from build123d import *

# Parameters (mm, degrees)
BOSS_EXTRUDE2_DEPTH  = 14.375
M4_CLEARANCE_HOLE2_D = 4.5
CUT_EXTRUDE1_START   = -5
SKETCH10_R           = 4.25
CUT_EXTRUDE1_DEPTH   = 30
M4_CLEARANCE_HOLE3_D = 4.5
CUT_EXTRUDE2_START   = -5
SKETCH14_R           = 4.25
CUT_EXTRUDE2_DEPTH   = 30
CHAMFER1_SIZE        = 1
FILLET2_R            = 1


with BuildPart() as part:
    # Sketch5 → Boss-Extrude2 (new, symmetric)
    with BuildSketch(Plane.XY):
        Polygon((0, 0), (0, 25.4), (-50.8, 0), align=None)
    extrude(amount=BOSS_EXTRUDE2_DEPTH, both=True)

    # M4 Clearance Hole2 (through all)
    with Locations(Plane(origin=(0, 0, 0), x_dir=(0, 0, -1), z_dir=(1, 0, 0))):
        with Locations((0, 12.390983006)):
            Hole(M4_CLEARANCE_HOLE2_D / 2)

    # Sketch10 → Cut-Extrude1 (cut)
    with BuildSketch(Plane(origin=(0, 0, 0), x_dir=(0, 0, -1), z_dir=(1, 0, 0)).offset(CUT_EXTRUDE1_START)):
        with Locations((0, 12.390983006)):
            Circle(SKETCH10_R)
    extrude(amount=-CUT_EXTRUDE1_DEPTH, mode=Mode.SUBTRACT)

    # M4 Clearance Hole3 (through all)
    with Locations(Plane(origin=(0, 0, 0), x_dir=(-1, 0, 0), z_dir=(0, -1, 0))):
        with Locations((25.4, 0)):
            Hole(M4_CLEARANCE_HOLE3_D / 2)

    # Sketch14 → Cut-Extrude2 (cut)
    with BuildSketch(Plane.XZ.offset(CUT_EXTRUDE2_START)):
        with Locations(Location((-25.4, 0, 0), (0, 0, 270))):
            Circle(SKETCH14_R)
    extrude(amount=-CUT_EXTRUDE2_DEPTH, mode=Mode.SUBTRACT)

    # Chamfer1
    chamfer1_edges = [part.edges().sort_by_distance(p)[0] for p in [
        (0, 0, 0),
    ]]
    chamfer(chamfer1_edges, length=CHAMFER1_SIZE)

    # Fillet2
    fillet2_edges = [part.edges().sort_by_distance(p)[0] for p in [
        (-25.4, 12.7, 14.375),
        (-25.4, 12.7, -14.375),
        (-25.9, 0, -14.375),
        (-25.9, 0, 14.375),
        (0, 13.2, -14.375),
        (0, 13.2, 14.375),
        (-0.5, 0.5, -14.375),
        (-0.5, 0.5, 14.375),
        (-50.8, 0, 0),
        (0, 25.4, 0),
    ]]
    fillet(fillet2_edges, radius=FILLET2_R)


solid = part.part
CAD build for the part. Positions are in the model's coordinates, mm. A direction names the side the tool comes from. Coordinates: 2 decimals unless noted, no trailing zeros. Loops run counter-clockwise (first coordinate to the right, second up) from the corner with the lowest first, then second, coordinate; pieces in that order, holes last. Notation, with made-up numbers: (88.5, -23.5) - (108.5, -23.5) arc R25 cw to (108.5, -7.5) - close; hole circle Ø2 at (79.5, 62). An arc over 180 degrees is marked (long way). Use one line per item in the form item = value. Start each with the question number.
1) Two-plate mould, pull along Y, no slides. Class faces 1 (the face through (-2.535, 10.395, 1.038)), 2 (the face through (-0.5, 0.5, 0.2)), 3 (the face through (-24.41, 12.86, -14.09)), 4 (the face through (-5, 11, -2)): +Y half, -Y half, draft (parallel to the pull), parting line (faces both ways), or undercut.
2) Band-saw the part on A-A (z = 1.25). Give the cut face in (x, y), and give its area (3 significant figures).
3) Flat gauge pins, fed straight in: pin 1 (1 mm diameter, centred on x = -21, y = 16.5, fed in from -Z); pin 2 (7 mm diameter, centred on y = 12.39, z = 0, fed in from -X); pin 3 (6 mm diameter, centred on y = 9, z = -9, fed in from -X); pin 4 (2.5 mm diameter, centred on x = -25.5, z = 1.5, fed in from +Y). Where does each tip first touch, or does it go through?
4) Band-saw the part on B-B (z = 5). Give the cut face in (x, y).
5) Tool access for faces 5 (the face through (-12.79, 8.24, 0.92)), 6 (the face through (-23.46, 0.3, 14.09)), 7 (the face through (-22.528, 7.823, 3.132)): list every direction of +Z, -Z, +X, -X, +Y, -Y with a clear straight run to the whole face (end or side of a thin tool).
6) Drill centre lines: L1, parallel to Y at x = -3.25, z = 0 (3 decimals); L2, parallel to Z at x = -25.4, y = 2.85 (3 decimals); L3, parallel to X at y = 6.5, z = 0. Where is each one in solid material? Low to high. Write a range as from..to.
Check values:
q1.face_1 = undercut
q1.face_2 = -Y half
q1.face_3 = +Y half
q1.face_4 = undercut
q2.outline = (-47.01, 1.89) arc R1 ccw to (-46.56, 0) - (-27.27, 0) - (-27.27, 5) - (-29.46, 5) - (-29.46, 8.33) - (-34.14, 8.33) - close; (-23.53, 0) - (-1, 0) - (0, 1) - (0, 10.52) - (-5, 10.52) - (-5, 8.33) - (-21.34, 8.33) - (-21.34, 5) - (-23.53, 5) - close; (-17.89, 16.45) - (-5, 16.45) - (-5, 14.26) - (0, 14.26) - (0, 23.78) arc R1 ccw to (-1.45, 24.68) - close
q2.area = 406 mm2
q3.pin_1 = through
q3.pin_2 = -5
q3.pin_3 = -38.8
q3.pin_4 = 5
q4.outline = (-47.01, 1.89) arc R1 ccw to (-46.56, 0) - (-1, 0) - (0, 1) - (0, 23.78) arc R1 ccw to (-1.45, 24.68) - close
q5.face_5 = -X
q5.face_6 = +Z, +X, -X, -Y
q5.face_7 = +Y
q6.L1 = 0..10.141, 14.641..23.775
q6.L2 = -14.375..-2.25, 2.25..14.375
q6.L3 = -37.8..-29.65, -21.15..0
